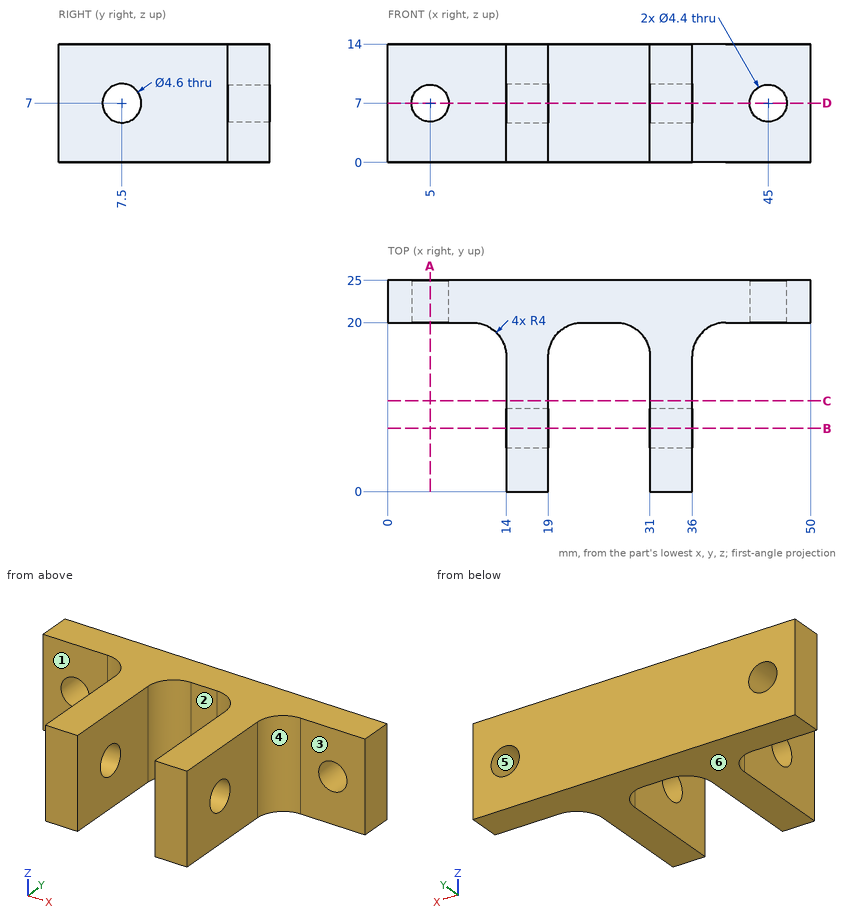
For this review, use the dimensioned drawing (mm, ordinates from the lowest corner) and the shaded views. A direction names the side the tool comes from. Give positions to 0.01 mm unless a question says otherwise; leave off trailing zeros. Order: outer loops, then holes, each group sorted by start corner. A loop starts at its lowest first (then second) coordinate and runs counter-clockwise, first axis right, second up. Notation, with made-up numbers: M -10.5,9.5 L 14.5,9.5 A20 cw 14.5,18.5 Z; hole C 51,63.5 d8. An arc over 180 degrees is marked long. Use one line per item in the form item = value. Start each with the question number.
Item 1: We need section C-C on y = 10.75. Give the boundary of the cut face in (x, z).
Item 2: To check wall thickness, follow line 1 along X through (y, z) = (12.25, 2.25); line 2 along Z through (x, y) = (16.1, 7.5); line 3 along Z through (x, y) = (45, 23.15). State the ranges of each line that lie inside material, in increasing order. Write a range as from..to.
Item 3: For the marked faces 1, 2 and 3, list the 3-axis set-ups (+Z, -Z, +X, -X, +Y, -Y) from which the entire face can be reached by the end or side of a thin tool; tool diameter is ignored.
Item 4: Insertion check: pin 1 Ø5 at (y, z) = (9.5, 3) entering from -X; pin 2 Ø1 at (y, z) = (12.5, 7.5) entering from +X; pin 3 Ø5 at (x, z) = (5, 7) entering from -Y. Each pin has a flat end and moves straight along its axis. Give the tip position at first contact, or say it passes through.
Item 5: We need section A-A on x = 5. Give the boundary of the cut face in (y, z), plus the area to 3 significant figures.
Item 6: We need section B-B on y = 7.5. Give the boundary of the cut face in (x, z), plus the area to 3 significant figures.
Item 7: The part is to be moulded in two halves that separate along Z. For the marked faces 4, 5 and 6, say which applies: pulls with the +Z half, pulls with the -Z half, needs draft (parallel to the pull), parting line crosses it, or undercut.
Item 8: We need section D-D on z = 7. Give the number of separate pieces and of enclosed holes in the cut face, plus the area to 3 significant figures.
Completed:
q1.outline = M 14,0 L 19,0 L 19,14 L 14,14 Z; M 31,0 L 36,0 L 36,14 L 31,14 Z
q2.line_1 = 14..19, 31..36
q2.line_2 = 0..4.7, 9.3..14
q2.line_3 = 0..4.8, 9.2..14
q3.face_1 = +Z, -Z, -X, -Y
q3.face_2 = +Z, -Z, -Y
q3.face_3 = +Z, -Z, +X, -Y
q4.pin_1 = 14
q4.pin_2 = 36
q4.pin_3 = 20
q5.outline = M 20,0 L 25,0 L 25,4.8 L 20,4.8 Z; M 20,9.2 L 25,9.2 L 25,14 L 20,14 Z
q5.area = 48.0 mm²
q6.outline = M 14,0 L 19,0 L 19,4.7 L 14,4.7 Z; M 14,9.3 L 19,9.3 L 19,14 L 14,14 Z; M 31,0 L 36,0 L 36,4.7 L 31,4.7 Z; M 31,9.3 L 36,9.3 L 36,14 L 31,14 Z
q6.area = 94.0 mm²
q7.face_4 = needs draft
q7.face_5 = undercut
q7.face_6 = pulls with the -Z half
q8.separate_pieces = 5
q8.enclosed_holes = 0
q8.area = 374 mm²
